Design review of the part built by this model. Coordinates are the model's own, in mm. A direction names the side the tool comes from. Round coordinates to 2 decimals unless told otherwise and drop trailing zeros. Loops run counter-clockwise (first coordinate to the right, second up) from the corner with the lowest first, then second, coordinate; pieces in that order, holes last. Notation, with made-up numbers: M 37.5,-12.75 L 61.5,-12.75 A26 cw 61.5,6.25 Z; hole C -32.75,-40 d10. An arc over 180 degrees is marked long. Use a Markdown table: item, result.
from build123d import *

# Parameters (mm, degrees)
SKETCH_1_R           = 21
EXTRUDE_3_DEPTH      = 6.3
EXTRUDE_3_2_DEPTH    = 6.3
SKETCH_3_R           = 6.25
EXTRUDE_4_DEPTH      = 33
EXTRUDE_5_DEPTH      = 140
EXTRUDE_5_DEPTH_BACK = 110
SKETCH_4_R           = 11
SKETCH_5_R           = 3
CUT_EXTRUDE_1_DEPTH  = 10


with BuildPart() as part:
    # Sketch 1 → Extrude 3 (new body)
    with BuildSketch(Plane.XY):
        with Locations((-64.202643172, 0)):
            Circle(SKETCH_1_R)
    extrude(amount=EXTRUDE_3_DEPTH)



with BuildPart() as body_2:
    # Sketch 1 → Extrude 3 2 (new body)
    with BuildSketch(Plane.XY):
        with Locations((95.797356828, 0)):
            Circle(SKETCH_1_R)
    extrude(amount=EXTRUDE_3_2_DEPTH)


with BuildPart() as part_1:
    add(part.part)

    add(body_2.part)  # Extrude 4 merges body 2
    # Sketch 3 → Extrude 4 (add)
    with BuildSketch(Plane.XY):
        with Locations((-64.202643172, 0)):
            Circle(SKETCH_3_R)
        with Locations((95.797356828, 0)):
            Circle(SKETCH_3_R)
    extrude(amount=EXTRUDE_4_DEPTH)

    # Sketch 4 → Extrude 5 (add, two sides: drawn at the far end of the back side and taken through both)
    with BuildSketch(Plane(origin=(0, 0, 0), x_dir=(0, 0, -1), z_dir=(1, 0, 0)).offset(-EXTRUDE_5_DEPTH_BACK)):
        with Locations((-42.051933495, 0)):
            Circle(SKETCH_4_R)
    extrude(amount=EXTRUDE_5_DEPTH + EXTRUDE_5_DEPTH_BACK)

    # Sketch 5 → Cut-Extrude 1 (cut)
    with BuildSketch(Plane.XY.offset(6.3)):
        with Locations((-64.202643172, 14.5)):
            Circle(SKETCH_5_R)
        with Locations((-64.202643172, -14.5)):
            Circle(SKETCH_5_R)
        with Locations((95.797356828, 14.5)):
            Circle(SKETCH_5_R)
        with Locations((95.797356828, -14.5)):
            Circle(SKETCH_5_R)
    extrude(amount=-CUT_EXTRUDE_1_DEPTH, mode=Mode.SUBTRACT)


solid = part_1.part
1. The part is to be moulded in two halves that separate along Y. For faces 1 (the face through (90.8, -4.4, 6.3)), 2 (the face through (13.25, 0.48, 53.04)), 3 (the face through (-61.43, -15.65, 3.19)), say which applies: pulls with the +Y half, pulls with the -Y half, needs draft (parallel to the pull), parting line crosses it, or undercut.
Check values:
| item | result |
|---|---|
| face 1 | needs draft |
| face 2 | parting line crosses it |
| face 3 | undercut |
2. Machinability: for faces 4 (the face through (-44.172, 6.308, 3.106)), 5 (the face through (98.57, -15.65, 3.19)), 6 (the face through (-60, 5, 6.3)), which of the approach directions +Z, -Z, +X, -X, +Y, -Y give a long, thin tool a straight path to every point of the face, cutting with its end or side? Answer none if there is none.
Check values:
| item | result |
|---|---|
| face 4 | -Z |
| face 5 | +Z, -Z |
| face 6 | none |
3. Insertion check: pin 1 (10 mm diameter, centred on x = 43.5, y = 7, fed in from +Z); pin 2 (5 mm diameter, centred on x = -23.5, y = -6, fed in from -Z); pin 3 (6 mm diameter, centred on x = -51, z = 45.5, fed in from +Y). Each pin has a flat end and moves straight along its axis. Give the tip position at first contact, or say it passes through.
Check values:
| item | result |
|---|---|
| pin 1 | stops at z = 52.87 |
| pin 2 | stops at z = 31.62 |
| pin 3 | stops at y = 10.99 |
4. Wall thickness on line 1 along X through (y, z) = (-14, 3); line 2 along X through (y, z) = (13, 6); line 3 along Z through (x, y) = (-61, 19.5): over which ranges is each line inside the solid? List them lowest first. Write a range as from..to.
Check values:
| item | result |
|---|---|
| line 1 | x = -79.86..-67.16, -61.24..-48.55, 80.14..92.84, 98.76..111.45 |
| line 2 | x = -80.7..-66.8, -61.6..-47.71, 79.3..93.2, 98.4..112.29 |
| line 3 | z = 0..6.3 |
5. Take a section at B-B on y = 0. Give the boundary of the cut face in (x, z), and give its area (3 significant figures).
Check values:
| item | result |
|---|---|
| outline | M -110,31.05 L -70.45,31.05 L -70.45,6.3 L -85.2,6.3 L -85.2,0 L -43.2,0 L -43.2,6.3 L -57.95,6.3 L -57.95,31.05 L 89.55,31.05 L 89.55,6.3 L 74.8,6.3 L 74.8,0 L 116.8,0 L 116.8,6.3 L 102.05,6.3 L 102.05,31.05 L 140,31.05 L 140,53.05 L -110,53.05 Z |
| area | 6,650 mm² |
6. Take a section at C-C on y = 14.5. Give the boundary of the cut face in (x, z), and give its area (3 significant figures).
Check values:
| item | result |
|---|---|
| outline | M -79.39,0 L -67.2,0 L -67.2,6.3 L -79.39,6.3 Z; M -61.2,0 L -49.01,0 L -49.01,6.3 L -61.2,6.3 Z; M 80.61,0 L 92.8,0 L 92.8,6.3 L 80.61,6.3 Z; M 98.8,0 L 110.99,0 L 110.99,6.3 L 98.8,6.3 Z |
| area | 307 mm² |
7. Take a section at D-D on z = 17. Give the boundary of the cut face in (x, y).
Check values:
| item | result |
|---|---|
| outline | C -64.2,0 d12.5; C 95.8,0 d12.5 |
8. Take a section at A-A on x = -64.5. Give the boundary of the cut face in (y, z), and give its area (3 significant figures).
Check values:
| item | result |
|---|---|
| outline | M -21,0 L -17.49,0 L -17.49,6.3 L -21,6.3 Z; M -11.51,0 L 11.51,0 L 11.51,6.3 L 6.24,6.3 L 6.24,33 A11 ccw long -6.24,33 L -6.24,6.3 L -11.51,6.3 Z; M 17.49,0 L 21,0 L 21,6.3 L 17.49,6.3 Z |
| area | 886 mm² |
